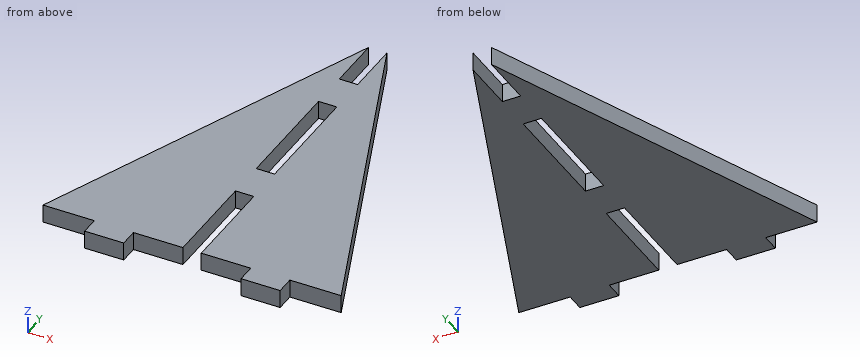
```python
from build123d import *

# Parameters (mm, degrees)
F1_DEPTH = 2.9718
F2_W     = 2.9718
F2_H     = 19.05
F2_H_2   = 25.4
F3_DEPTH = 25.4
F4_W     = 8.0391
F4_H     = 2.9718
F4_W_2   = 12.7
F5_DEPTH = 25.4


with BuildPart() as f1:
    # F0 (on Top) → F1 (new body)
    with BuildSketch(Plane.XY):
        Polygon((25.4, 0), (0, 63.5), (-25.4, 0), align=None)
    extrude(amount=F1_DEPTH)

    # F2 (on face) → F3 (cut)
    with BuildSketch(Plane.XY.offset(2.9718)):
        with Locations((0, 9.525)):
            Rectangle(F2_W, F2_H)
        with Locations((0, 34.925)):
            Rectangle(F2_W, F2_H)
        with Locations((0, 63.5)):
            Rectangle(F2_W, F2_H_2)
    extrude(amount=-F3_DEPTH, mode=Mode.SUBTRACT)

    # F4 (on face) → F5 (cut)
    with BuildSketch(Plane.XY.offset(2.9718)):
        with Locations((-5.50545, 1.4859)):
            Rectangle(F4_W, F4_H)
        with Locations((-22.225, 1.4859)):
            Rectangle(F4_W_2, F4_H)
        with Locations((5.50545, 1.4859)):
            Rectangle(F4_W, F4_H)
        with Locations((22.225, 1.4859)):
            Rectangle(F4_W_2, F4_H)
    extrude(amount=-F5_DEPTH, mode=Mode.SUBTRACT)


solid = f1.part
```
Input: part model. Units: mm. Frame: model coordinates. Give positions to 0.01 mm unless a question says otherwise; leave off trailing zeros. Loops run counter-clockwise (first coordinate to the right, second up) from the corner with the lowest first, then second, coordinate; pieces in that order, holes last. Notation, with made-up numbers: (76.5, -16) -> (88.5, -16) arc R31 ccw to (88.5, 16) -> close; hole circle Ø10 at (17, 47.5). An arc over 180 degrees is marked (long way). Use a Markdown table: item, result.
Q1. Ray query, probe 1 along Y at (x, z) = (0.5, 1.4); probe 2 along X at (y, z) = (51, 0.35); probe 3 along X at (y, z) = (7, 2.35). Return the intervals inside material, ascending. Write a range as from..to.
Entries:
| item | result |
|---|---|
| probe 1 | y = 19.05..25.4, 44.45..50.8 |
| probe 2 | x = -5..-1.49, 1.49..5 |
| probe 3 | x = -22.6..-1.49, 1.49..22.6 |
Q2. Section query C-C, the plane x = 0.5. Return the cut outline in (y, z), plus the area to 3 significant figures.
Entries:
| item | result |
|---|---|
| outline | (19.05, 0) -> (25.4, 0) -> (25.4, 2.97) -> (19.05, 2.97) -> close; (44.45, 0) -> (50.8, 0) -> (50.8, 2.97) -> (44.45, 2.97) -> close |
| area | 37.7 mm² |
Q3. First-contact query: P1, Ø1.5, axis at x = 19.5, z = 1, coming from the -Y side; P2, Ø1.5, axis at y = 53, z = 2.5, coming from the -X side; P3, Ø1.5, axis at y = 34, z = 2, coming from the -X side. Flat tips, straight axial feed; report the tip coordinate or a pass-through.
Entries:
| item | result |
|---|---|
| P1 | stops at y = 2.97 |
| P2 | stops at x = -4.5 |
| P3 | stops at x = -12.1 |
Q4. Section query D-D, the plane x = -20. Return the cut outline in (y, z).
Entries:
| item | result |
|---|---|
| outline | (2.97, 0) -> (13.5, 0) -> (13.5, 2.97) -> (2.97, 2.97) -> close |
Q5. Section query A-A, the plane z = 1.55. Return the cut outline in (x, y) (3 decimals).
Entries:
| item | result |
|---|---|
| outline | (-24.211, 2.972) -> (-15.875, 2.972) -> (-15.875, 0) -> (-9.525, 0) -> (-9.525, 2.972) -> (-1.486, 2.972) -> (-1.486, 19.05) -> (1.486, 19.05) -> (1.486, 2.972) -> (9.525, 2.972) -> (9.525, 0) -> (15.875, 0) -> (15.875, 2.972) -> (24.211, 2.972) -> (1.486, 59.785) -> (1.486, 50.8) -> (-1.486, 50.8) -> (-1.486, 59.785) -> close; hole (-1.486, 25.4) -> (1.486, 25.4) -> (1.486, 44.45) -> (-1.486, 44.45) -> close |
Q6. Section query B-B, the plane y = 55. Return the cut outline in (x, z).
Entries:
| item | result |
|---|---|
| outline | (-3.4, 0) -> (-1.49, 0) -> (-1.49, 2.97) -> (-3.4, 2.97) -> close; (1.49, 0) -> (3.4, 0) -> (3.4, 2.97) -> (1.49, 2.97) -> close |
